Source: CAD feature listing. Evaluate the final solid. Frame: model axes, mm. Face numbers are marked on the shaded views. A direction names the side the tool comes from. Round coordinates to 2 decimals unless told otherwise and drop trailing zeros. Order: outer loops, then holes, each group sorted by start corner. A loop starts at its lowest first (then second) coordinate and runs counter-clockwise, first axis right, second up. Notation, with made-up numbers: (-36.5, -17) -> (9.5, -17) arc R28 cw to (9.5, 17) -> close; hole circle Ø11 at (-17.75, 47.25). An arc over 180 degrees is marked (long way). One line per item, written item: value. Start each with the question number.
1) Section C-C (y = 1.45). Return the cut outline in (x, z).
2) Reachability of the marked faces 4, 5 and 6 from +Z, -Z, +X, -X, +Y, -Y: full face, straight path, thin tool, end or side. Return the list, or none.
3) Section A-A (x = 0). Return the cut outline in (y, z), and give its area (3 significant figures).
4) Section B-B (z = 0). Return the cut outline in (x, y).
5) Ray query, L1, parallel to X at y = 2.95, z = 0; L2, parallel to X at y = 1.1, z = 0; L3, parallel to Y at x = 3.5, z = 3. Return the intervals inside material, ascending.
6) Mould query, pull axis X, two halves, no side actions, for the marked faces 1, 2 and 3. Classes: pulls with the +X half, pulls with the -X half, needs draft (parallel to the pull), parting line crosses it, or undercut.
7) Pin query (flat end, axial travel): P1, Ø2, axis at x = -1.5, y = 4, coming from the -Z side; P2, Ø2, axis at y = 1, z = -0.5, coming from the +X side; P3, Ø1.5, axis at x = 3, y = 1.5, coming from the -Z side; P4, Ø2, axis at y = 1, z = 2.5, coming from the -X side. Return the tip coordinate at first contact, or that it passes through.
8) Section D-D (y = 4.65). Return the cut outline in (x, z).
```python
from build123d import *

# Parameters (mm, degrees)
SKETCH1_R           = 3.5
SKETCH1_R_2         = 2.55
BOSS_EXTRUDE1_DEPTH = 4
SKETCH2_R           = 3.5
BOSS_EXTRUDE2_DEPTH = 2
SKETCH4_R           = 5
SKETCH4_R_2         = 3.5
BOSS_EXTRUDE3_DEPTH = 2


with BuildPart() as part:
    # Sketch1 → Boss-Extrude1 (new body)
    with BuildSketch(Plane(origin=(0, 0, 0), x_dir=(1, 0, 0), z_dir=(0, 1, 0))):
        with Locations(Location((0, 0, 0), (0, 0, 270))):
            Circle(SKETCH1_R)
        with Locations(Location((0, 0, 0), (0, 0, 270))):
            Circle(SKETCH1_R_2, mode=Mode.SUBTRACT)
    extrude(amount=BOSS_EXTRUDE1_DEPTH)

    # Sketch2 → Boss-Extrude2 (add)
    with BuildSketch(Plane(origin=(0, 4, 0), x_dir=(1, 0, 0), z_dir=(0, 1, 0))):
        with Locations(Location((0, 0, 0), (0, 0, 270))):
            Circle(SKETCH2_R)
    extrude(amount=BOSS_EXTRUDE2_DEPTH)

    # Sketch4 → Boss-Extrude3 (add)
    with BuildSketch(Plane(origin=(0, 0, 0), x_dir=(-1, 0, 0), z_dir=(0, -1, 0))):
        with Locations(Location((0, 0, 0), (0, 0, 90))):
            Circle(SKETCH4_R)
        with Locations(Location((0, 0, 0), (0, 0, 90))):
            Circle(SKETCH4_R_2, mode=Mode.SUBTRACT)
    extrude(amount=-BOSS_EXTRUDE3_DEPTH)


solid = part.part
```
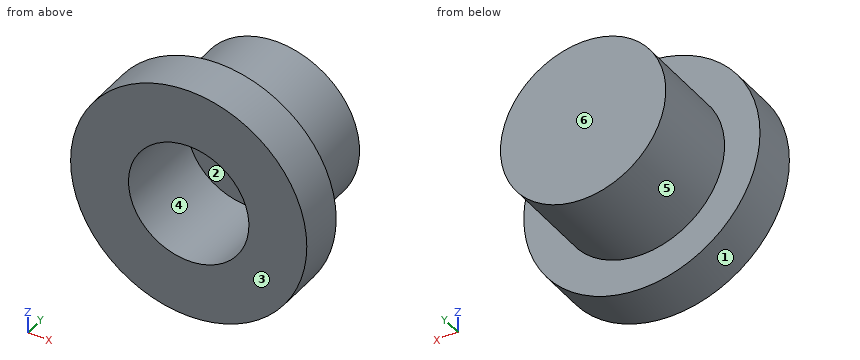
Findings:
1. outline: circle Ø10 at (0, 0); hole circle Ø5.1 at (0, 0)
2. face 4: -Y
2. face 5: +Y
2. face 6: +Z, -Z, +X, -X, +Y
3. outline: (0, -5) -> (2, -5) -> (2, -3.5) -> (6, -3.5) -> (6, 3.5) -> (2, 3.5) -> (2, 5) -> (0, 5) -> (0, 2.55) -> (4, 2.55) -> (4, -2.55) -> (0, -2.55) -> close
3. area: 27.6 mm2
4. outline: (-5, 0) -> (-2.55, 0) -> (-2.55, 4) -> (2.55, 4) -> (2.55, 0) -> (5, 0) -> (5, 2) -> (3.5, 2) -> (3.5, 6) -> (-3.5, 6) -> (-3.5, 2) -> (-5, 2) -> close
5. L1: -3.5 to -2.55, 2.55 to 3.5
5. L2: -5 to -2.55, 2.55 to 5
5. L3: 0 to 2
6. face 1: parting line crosses it
6. face 2: undercut
6. face 3: needs draft
7. P1: z = -3.46
7. P2: x = 5
7. P3: z = -4.47
7. P4: x = -4.77
8. outline: circle Ø7 at (0, 0)
